Autodesk Inventor part; units mm, degrees
ref_plane "YZ Plane" through (0, 0, 0) normal (1, 0, 0) x (0, 1, 0)
ref_plane "XZ Plane" through (0, 0, 0) normal (0, 1, 0) x (-1, 0, 0)
ref_plane "XY Plane" through (0, 0, 0) normal (0, 0, 1) x (1, 0, 0)
sketch "Skizze1" plane through (0, 0, 0) normal (0, 0, 1) x (1, 0, 0)
  line L0 (0, -5) -> (0, 5) construction
  line L1 (2.5, -5) -> (2.5, 5)
  line L2 (-2.5, 5) -> (-2.5, -5)
  arc A0 (-2.5, -5) -> (2.5, -5) centre (0, -5) ccw
  arc A1 (2.5, 5) -> (-2.5, 5) centre (0, 5) ccw
  point P0 (0, 0)
  dimension "d0" = 5
  dimension "d1" = 10
extrude "Extrusion1" add sketch "Skizze1" along normal blind 1.4
sketch "Skizze2" plane through (0, 0, 1.4) normal (0, 0, 1) x (1, 0, 0)
  line L0 (2.5, -5) -> (2.5, 5)
  arc A0 (2.5, 5) -> (-2.5, 5) centre (0, 5) ccw
  line L1 (-2.5, 5) -> (-2.5, -5)
  arc A1 (-2.5, -5) -> (2.5, -5) centre (0, -5) ccw
  line L2 (-2.5, 5) -> (-2.5, -5)
  line L3 (-2.5, 5) -> (2.5, 5)
  line L4 (2.5, -5) -> (2.5, 5)
  line L5 (2.5, -5) -> (-2.5, -5)
  arc A2 (2.5, 5) -> (-2.5, 5) centre (0, 5) ccw
  arc A3 (-2.5, -5) -> (2.5, -5) centre (0, -5) ccw
  line L6 (-2.5, 3.55) -> (2.5, 3.55)
  line L7 (2.5, 3.55) -> (2.5, 2.15)
  line L8 (2.5, 2.15) -> (-2.5, 2.15)
  line L9 (-2.5, 2.15) -> (-2.5, 3.55)
  line L10 (2.5, 0.7) -> (-2.5, 0.7)
  line L11 (-2.5, 0.7) -> (-2.5, -0.7)
  line L12 (-2.5, -0.7) -> (2.5, -0.7)
  line L13 (2.5, -0.7) -> (2.5, 0.7)
  line L14 (-2.5, -2.15) -> (2.5, -2.15)
  line L15 (2.5, -2.15) -> (2.5, -3.55)
  line L16 (2.5, -3.55) -> (-2.5, -3.55)
  line L17 (-2.5, -3.55) -> (-2.5, -2.15)
  line L18 (-3.5, 0) -> (3.5, 0)
  line L19 (-2.5, 2.85) -> (2.5, 2.85) construction
  point P0 (0, 0)
  dimension "d4" = 1.4
  dimension "d5" = 1.4
extrude "Extrusion2" add sketch "Skizze2" along normal blind 0.8 contours A1 L5 | L16 L1 L14 L0 | L12 L1 L18 L0 | L18 L1 L10 L0 | L8 L1 L6 L0 | L3 A0
equation "\"d5\" = d4"
properties part number "Dribblerdaempfer Unten" material "Gummi, Silikon"
Can you work these out from the model? Positions are in its coordinate system, mm. A direction names the side the tool comes from. Round coordinates to 2 decimals unless told otherwise and drop trailing zeros. Loops run counter-clockwise (first coordinate to the right, second up) from the corner with the lowest first, then second, coordinate; pieces in that order, holes last. Notation, with made-up numbers: M 81.5,65.25 L 118.5,65.25 A20 ccw 118.5,87.25 Z; hole C -16.5,36 d3. An arc over 180 degrees is marked long. Write item = value, one per line. Start each with the question number.
(1) If we mould it in two halves opening along Y, with no side actions, what happens to faces 1 (the face through (0, 2.15, 2)), 2 (the face through (-2.5, 0, 1)), 3 (the face through (0.1, -7.5, 1.1))? For each: released by +Y, released by -Y, zero draft, split by the parting line, or undercut.
(2) Suppose I cut it at D-D on z = 1.2. Write out the boundary of the cut face in (x, y), plus the area to 3 significant figures.
(3) Suppose I cut it at C-C on y = 4. Write out the boundary of the cut face in (x, z), plus the area to 3 significant figures.
(4) I'm going to push flat-ended pins straight in: P1, Ø1.2, axis at x = 1, y = 1.5, coming from the +Z side; P2, Ø0.9, axis at x = 1, z = 2, coming from the -Y side. Where does each tip first touch, or does it pass through?
(5) Suppose I cut it at A-A on z = 2. Write out the boundary of the cut face in (x, y).
(6) Suppose I cut it at B-B on x = 0. Write out the boundary of the cut face in (y, z), plus the area to 3 significant figures.
(7) Which directions (+Z, -Z, +X, -X, +Y, -Y) give clear straight access to the entire face, cutting with the end or side of a thin tool? Please do faces 4 (the face through (0, -3.55, 2)), 5 (the face through (0, 6, 2.2)).
(8) I need wall thicknesses on line 1 along Y through (x, z) = (0.1, 1.8); line 2 along Y through (x, z) = (-0.65, 2.1); line 3 along Z through (x, y) = (1.55, -4.5). Which ranges of each line are inside material? Lowest first, please.
Answer block:
q1.face_1 = undercut
q1.face_2 = zero draft
q1.face_3 = released by -Y
q2.outline = M -2.5,-5 A2.5 ccw 2.5,-5 L 2.5,5 A2.5 ccw -2.5,5 Z
q2.area = 69.6 mm²
q3.outline = M -2.5,0 L 2.5,0 L 2.5,1.4 L -2.5,1.4 Z
q3.area = 7.00 mm²
q4.P1 = 1.4
q4.P2 = -7.44
q5.outline = M -2.5,-5 A2.5 ccw 2.5,-5 Z; M -2.5,-3.55 L 2.5,-3.55 L 2.5,-2.15 L -2.5,-2.15 Z; M -2.5,-0.7 L 2.5,-0.7 L 2.5,0.7 L -2.5,0.7 Z; M -2.5,2.15 L 2.5,2.15 L 2.5,3.55 L -2.5,3.55 Z; M -2.5,5 L 2.5,5 A2.5 ccw Z
q6.outline = M -7.5,0 L 7.5,0 L 7.5,2.2 L 5,2.2 L 5,1.4 L 3.55,1.4 L 3.55,2.2 L 2.15,2.2 L 2.15,1.4 L 0.7,1.4 L 0.7,2.2 L -0.7,2.2 L -0.7,1.4 L -2.15,1.4 L -2.15,2.2 L -3.55,2.2 L -3.55,1.4 L -5,1.4 L -5,2.2 L -7.5,2.2 Z
q6.area = 28.4 mm²
q7.face_4 = +Z, +X, -X
q7.face_5 = +Z, +X, -X, +Y, -Y
q8.line_1 = -7.5 to -5, -3.55 to -2.15, -0.7 to 0.7, 2.15 to 3.55, 5 to 7.5
q8.line_2 = -7.41 to -5, -3.55 to -2.15, -0.7 to 0.7, 2.15 to 3.55, 5 to 7.41
q8.line_3 = 0 to 1.4
